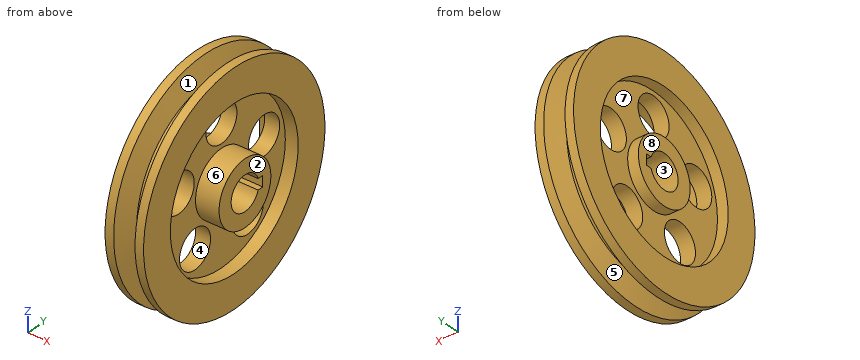
```python
from build123d import *

# Parameters (mm, degrees)
SKETCH_2_R        = 8
F_02_BORE_DEPTH   = 25
SKETCH_3_W        = 5
SKETCH_3_H        = 3.3
F_03_KEYWAY_DEPTH = 25
SKETCH_4_R        = 9
F_04_HOLE_0_DEPTH = 9
SKETCH_5_R        = 9
F_04_HOLE_1_DEPTH = 9
SKETCH_6_R        = 9
F_04_HOLE_2_DEPTH = 9
SKETCH_7_R        = 9
F_04_HOLE_3_DEPTH = 9
SKETCH_8_R        = 9
F_04_HOLE_4_DEPTH = 9


with BuildPart() as part:
    # 草图1 → 01_BODY (revolve)
    with BuildSketch(Plane.XY, mode=Mode.PRIVATE) as f_01_body_sk:
        Polygon((0, 0), (23, 0), (23, 15), (12, 15), (12, 37), (18, 37), (18, 52.5), (14, 52.5), (11.320508076, 42.5), (6.679491924, 42.5), (4, 52.5), (0, 52.5), (0, 37), (5, 37), (5, 15), (0, 15), align=None)
    revolve(f_01_body_sk.sketch.rotate(Axis((-5, 0, 0), (1, 0, 0)), 90), axis=Axis((-5, 0, 0), (1, 0, 0)))

    # 草图2 → 02_BORE (cut)
    with BuildSketch(Plane(origin=(-1, 0, 0), x_dir=(0, 0, -1), z_dir=(1, 0, 0))):
        with Locations(Location((0, 0, 0), (0, 0, 180))):
            Circle(SKETCH_2_R)
    extrude(amount=F_02_BORE_DEPTH, mode=Mode.SUBTRACT)

    # 草图3 → 03_KEYWAY (cut)
    with BuildSketch(Plane(origin=(-1, 0, 0), x_dir=(0, 0, -1), z_dir=(1, 0, 0))):
        with Locations((0, 8.65)):
            Rectangle(SKETCH_3_W, SKETCH_3_H)
    extrude(amount=F_03_KEYWAY_DEPTH, mode=Mode.SUBTRACT)

    # 草图4 → 04_HOLE_0 (cut)
    with BuildSketch(Plane(origin=(4, 0, 0), x_dir=(0, 0, -1), z_dir=(1, 0, 0))):
        with Locations(Location((-26, 0, 0), (0, 0, 180))):
            Circle(SKETCH_4_R)
    extrude(amount=F_04_HOLE_0_DEPTH, mode=Mode.SUBTRACT)

    # 草图5 → 04_HOLE_1 (cut)
    with BuildSketch(Plane(origin=(4, 0, 0), x_dir=(0, 0, -1), z_dir=(1, 0, 0))):
        with Locations(Location((-8.034441854, -24.727469424, 0), (0, 0, 180))):
            Circle(SKETCH_5_R)
    extrude(amount=F_04_HOLE_1_DEPTH, mode=Mode.SUBTRACT)

    # 草图6 → 04_HOLE_2 (cut)
    with BuildSketch(Plane(origin=(4, 0, 0), x_dir=(0, 0, -1), z_dir=(1, 0, 0))):
        with Locations(Location((21.034441854, -15.28241656, 0), (0, 0, 180))):
            Circle(SKETCH_6_R)
    extrude(amount=F_04_HOLE_2_DEPTH, mode=Mode.SUBTRACT)

    # 草图7 → 04_HOLE_3 (cut)
    with BuildSketch(Plane(origin=(4, 0, 0), x_dir=(0, 0, -1), z_dir=(1, 0, 0))):
        with Locations(Location((21.034441854, 15.28241656, 0), (0, 0, 180))):
            Circle(SKETCH_7_R)
    extrude(amount=F_04_HOLE_3_DEPTH, mode=Mode.SUBTRACT)

    # 草图8 → 04_HOLE_4 (cut)
    with BuildSketch(Plane(origin=(4, 0, 0), x_dir=(0, 0, -1), z_dir=(1, 0, 0))):
        with Locations(Location((-8.034441854, 24.727469424, 0), (0, 0, 180))):
            Circle(SKETCH_8_R)
    extrude(amount=F_04_HOLE_4_DEPTH, mode=Mode.SUBTRACT)


solid = part.part
```
Check sheet for the modelled part. Datum: model origin and axes. Units: mm. Face numbers are marked on the shaded views. A direction names the side the tool comes from. Round coordinates to 2 decimals unless told otherwise and drop trailing zeros.
1) Go/stop test with flat-tipped pins: pin 1 Ø6 at (x, z) = (13, 28) entering from +Y; pin 2 Ø1 at (y, z) = (-40.5, -6.5) entering from +X; pin 3 Ø1 at (x, y) = (17, 24) entering from +Z. Record where each tip stops, or that it passes through.
2) Section check A-A (z = 5). Give the number of separate pieces and of enclosed holes in the cut face, and give its area (3 significant figures).
3) Mould release check, pull along Z, two halves, no side actions. Record for the marked faces 1, 2 and 3: +Z half, -Z half, draft (parallel to the pull), parting line (faces both ways), or undercut.
4) Tool access check on the marked faces 4, 5, 6, 7 and 8. Record the directions out of +Z, -Z, +X, -X, +Y, -Y that give a thin tool (end or side, any length) a straight path to the whole face; none if there is none.
5) Scan lines: line 1 (Y direction, x = 2.1, z = 0); line 2 (Z direction, x = 16, y = 2.5); line 3 (Z direction, x = 7.5, y = 18). Record each from-to range of solid material in increasing order.
Result:
1. pin 1: stops at y = 46.07
1. pin 2: stops at x = 18
1. pin 3: stops at z = 46.95
2. separate pieces: 4
2. enclosed holes: 0
2. area: 856 mm2
3. face 1: parting line
3. face 2: draft
3. face 3: undercut
4. face 4: +X, -X
4. face 5: none
4. face 6: +X
4. face 7: -X
4. face 8: +Z, -Z, -X, +Y, -Y
5. line 1: y = -52.5 to -37, -15 to -8, 10.3 to 15, 37 to 52.5
5. line 2: z = -52.44 to -36.92, -14.79 to -7.6, 7.6 to 14.79, 36.92 to 52.44
5. line 3: z = -38.5 to -29.61, -12.45 to 2.06, 14.01 to 38.5
